Read the model definition and answer for the solid it produces. Units are mm, in the model's axes. A direction names the side the tool comes from. Coordinates: 2 decimals unless noted, no trailing zeros. Write each loop counter-clockwise with the first axis right and the second up, starting at its lowest first coordinate (ties: lowest second). Pieces come first, ordered by that corner, then holes. Notation, with made-up numbers: (48.25, -3) -> (90.25, -3) arc R18 ccw to (90.25, 3) -> close; hole circle Ø1 at (59.25, -24.5). An arc over 180 degrees is marked (long way). Write item = value, one per line. Start each with the question number.
1) Section B-B (z = 25.5) is taken. Count the separate pieces of the cut face and the enclosed holes in it, plus the area to 3 significant figures.
2) Section A-A (x = -6.5) is taken. Determine the outline of the cut face in (y, z), plus the area to 3 significant figures.
3) For a pull along Z with two mould halves and no side action, classify faces 6 (the face through (20.514, 15.136, 164.907)), 7 (the face through (0, -2, 10)), 8 (the face through (20.514, 16.424, 178.678)), 9 (the face through (9.25, 31.99, 138.16)) as released by +Z, released by -Z, zero draft, split by the parting line, or undercut.
4) Flat-ended cylindrical pins translate along their axes: pin 1 Ø2 at (x, z) = (-20, 9) entering from +Y; pin 2 Ø1 at (y, z) = (17, 173.5) entering from -X; pin 3 Ø2 at (x, z) = (-9, 95.5) entering from -Y; pin 4 Ø6 at (y, z) = (26.5, 143) entering from +X. Find the tip coordinate at first contact, or state that the pin passes through.
5) Find the intervals of material crossed by line 1 along X through (y, z) = (30.7, 42.55); line 2 along Y through (x, z) = (-12.5, 16); line 3 along X through (y, z) = (9.5, 15), in increasing order. Write a range as from..to.
6) A tool of negligible diameter and unlimited length cuts with its end or side. For faces 1 (the face through (-20.514, 12.916, 159.812)), 2 (the face through (22.27, 4.46, 199.87)), 3 (the face through (20.51, 20.11, 81.98)), 4 (the face through (20, 4, 204.877)), 5 (the face through (-7.38, 31.99, 55.43)), from which of +Z, -Z, +X, -X, +Y, -Y can it reach the whole face along a straight path? Write none if from no direction.
from build123d import *

# Parameters (mm, degrees)
SKETCH1_W                                 = 4
SKETCH1_H                                 = 1.4
SKETCH1_W_2                               = 39
SKETCH1_H_2                               = 2
SKETCH1_W_3                               = 2
SKETCH1_H_3                               = 27.8
SKETCH1_W_4                               = 19.5
BOSS_EXTRUDE1_DEPTH                       = 195
CUT_EXTRUDE1_DEPTH                        = 203.393181703
CUT_EXTRUDE1_DEPTH_BACK                   = 203.393181703
SKETCH2_W                                 = 191
SKETCH2_H                                 = 24
SKETCH3_W                                 = 29
SKETCH3_H                                 = 223
CUT_EXTRUDE2_DEPTH                        = 2
SKETCH5_W                                 = 45.8
SKETCH5_H                                 = 4
BOSS_EXTRUDE2_DEPTH                       = 2
SKETCH8_W                                 = 15
SKETCH8_H                                 = 8
BOSS_EXTRUDE4_DEPTH                       = 2
SKETCH9_W                                 = 15
SKETCH9_H                                 = 8
BOSS_EXTRUDE5_DEPTH                       = 2
BOSS_EXTRUDE6_DEPTH                       = 2
SKETCH6_W                                 = 45.8
SKETCH6_H                                 = 2.4
BOSS_EXTRUDE9_DEPTH                       = 19
SKETCH14_R                                = 4.7
SKETCH14_R_2                              = 1.6
CUT_EXTRUDE3_DEPTH                        = 19
TAP_DRILL_FOR_M3X0_5_TAP1_D               = 2.8
TAP_DRILL_FOR_M3X0_5_TAP1_DEPTH           = 10
TAP_DRILL_FOR_M3X0_5_TAP1_TIP             = 0.841204867
TAP_DRILL_FOR_M3X0_5_TAP1_ON_FACE_2_D     = 2.8
TAP_DRILL_FOR_M3X0_5_TAP1_ON_FACE_2_DEPTH = 10
TAP_DRILL_FOR_M3X0_5_TAP1_ON_FACE_2_TIP   = 0.841204867
TAP_DRILL_FOR_M3X0_5_TAP2_D               = 2.8
TAP_DRILL_FOR_M3X0_5_TAP2_DEPTH           = 10
TAP_DRILL_FOR_M3X0_5_TAP2_TIP             = 0.841204867
BOSS_EXTRUDE10_DEPTH                      = 2
BOSS_EXTRUDE11_START                      = -21.5
BOSS_EXTRUDE11_DEPTH                      = 43
BOSS_EXTRUDE12_DEPTH                      = 3
BOSS_EXTRUDE12_DEPTH_BACK                 = 1
SKETCH23_W                                = 36
SKETCH23_H                                = 20
FILLET3_R                                 = 3
FILLET4_R                                 = 3
FILLET5_R                                 = 3
FILLET6_R                                 = 3
CHAMFER3_SIZE                             = 8
CHAMFER3_SIZE_2                           = 1.410615846
BOSS_EXTRUDE14_DEPTH                      = 10
BOSS_EXTRUDE15_DEPTH                      = 10
FILLET7_R                                 = 2
CUT_EXTRUDE6_DEPTH                        = 10
CUT_EXTRUDE6_DEPTH_BACK                   = 10
SKETCH28_W                                = 29
SKETCH28_H                                = 20
CUT_EXTRUDE7_DEPTH                        = 2


# Read off the part's stored shape, not the designer's step: Boss-Extrude11
# Some blends are built 0.0001 mm under size
with BuildPart() as part:
    # Sketch1 → Boss-Extrude1 (new body)
    with BuildSketch(Plane.XY):
        Polygon((19.5, 1), (19.5, -1), (21.5, -1), (21.5, 5.2), (19.5, 5.2), (19.5, 3.8), align=None)
        with Locations((17.5, 4.5)):
            Rectangle(SKETCH1_W, SKETCH1_H)
        Rectangle(SKETCH1_W_2, SKETCH1_H_2)
        Polygon((-21.5, -1), (-19.5, -1), (-19.5, 1), (-19.5, 3.8), (-19.5, 5.2), (-21.5, 5.2), align=None)
        with Locations((-17.5, 4.5)):
            Rectangle(SKETCH1_W, SKETCH1_H)
        with Locations((20.5, 19.1)):
            Rectangle(SKETCH1_W_3, SKETCH1_H_3)
        with Locations((9.75, 32)):
            Rectangle(SKETCH1_W_4, SKETCH1_H_2)
        with Locations((-9.75, 32)):
            Rectangle(SKETCH1_W_4, SKETCH1_H_2)
        Polygon((-21.5, 33), (-21.5, 5.2), (-19.5, 5.2), (-19.5, 31), (-19.5, 33), align=None)
    extrude(amount=BOSS_EXTRUDE1_DEPTH)

    # Sketch2 → Cut-Extrude1 (cut, two sides: drawn at the far end of the back side and taken through both)
    with BuildSketch(Plane(origin=(21.5, 0, 0), x_dir=(0, 0, -1), z_dir=(1, 0, 0)).offset(-CUT_EXTRUDE1_DEPTH_BACK)):
        with Locations((-99.5, 19)):
            Rectangle(SKETCH2_W, SKETCH2_H)
    extrude(amount=CUT_EXTRUDE1_DEPTH + CUT_EXTRUDE1_DEPTH_BACK, mode=Mode.SUBTRACT)

    # Sketch3 → Cut-Extrude2 (cut)
    with BuildSketch(Plane(origin=(0, -1, 0), x_dir=(-1, 0, 0), z_dir=(0, -1, 0))):
        with Locations((0, -103.5)):
            Rectangle(SKETCH3_W, SKETCH3_H)
    extrude(amount=-CUT_EXTRUDE2_DEPTH, mode=Mode.SUBTRACT)

    # Sketch5 → Boss-Extrude2 (add)
    with BuildSketch(Plane(origin=(21.5, 0, 0), x_dir=(0, 0, -1), z_dir=(1, 0, 0))):
        with Locations((-22.9, 31)):
            Rectangle(SKETCH5_W, SKETCH5_H)
    extrude(amount=-BOSS_EXTRUDE2_DEPTH)

    # Sketch8 → Boss-Extrude4 (add)
    with BuildSketch(Plane(origin=(21.5, 0, 0), x_dir=(0, 0, -1), z_dir=(1, 0, 0))):
        with Locations((-11.5, 11)):
            Rectangle(SKETCH8_W, SKETCH8_H)
    extrude(amount=-BOSS_EXTRUDE4_DEPTH)

    # Sketch9 → Boss-Extrude5 (add)
    with BuildSketch(Plane.ZY.offset(21.5)):
        with Locations((11.5, 11)):
            Rectangle(SKETCH9_W, SKETCH9_H)
    extrude(amount=-BOSS_EXTRUDE5_DEPTH)

    # Sketch10 → Boss-Extrude6 (add)
    with BuildSketch(Plane.ZY.offset(21.5)):
        Polygon((4, 31), (146.749133454, 7), (195, 7), (52.250866546, 31), align=None)
        Polygon((195, 31), (52.250866546, 7), (4, 7), (146.749133454, 31), align=None)
    extrude(amount=-BOSS_EXTRUDE6_DEPTH)

    # Sketch6 → Boss-Extrude9 (add)
    with BuildSketch(Plane(origin=(21.5, 0, 0), x_dir=(0, 0, -1), z_dir=(1, 0, 0))):
        with Locations((-22.9, 30.2)):
            Rectangle(SKETCH6_W, SKETCH6_H)
    extrude(amount=BOSS_EXTRUDE9_DEPTH)

    # Sketch14 → Cut-Extrude3 (cut)
    with BuildSketch(Plane(origin=(0, 29, 0), x_dir=(-1, 0, 0), z_dir=(0, -1, 0))):
        with Locations(Location((-29.082681436, -25.05, 0), (0, 0, 90))):
            Circle(SKETCH14_R)
        with Locations(Location((-36.882681436, -42.55, 0), (0, 0, 90))):
            Circle(SKETCH14_R_2)
        with Locations(Location((-36.882681436, -7.55, 0), (0, 0, 90))):
            Circle(SKETCH14_R_2)
    extrude(amount=-CUT_EXTRUDE3_DEPTH, mode=Mode.SUBTRACT)

    # Tap Drill for M3x0.5 Tap1
    with Locations(Plane(origin=(-21.5, 9, 9.5), x_dir=(0, 0, -1), z_dir=(-1, 0, 0))):
        with Locations((0, 0)):
            Hole(TAP_DRILL_FOR_M3X0_5_TAP1_D / 2, depth=TAP_DRILL_FOR_M3X0_5_TAP1_DEPTH)
            with Locations((0, 0, -(TAP_DRILL_FOR_M3X0_5_TAP1_DEPTH + TAP_DRILL_FOR_M3X0_5_TAP1_TIP / 2))):  # 118° drill point
                Cone(0, TAP_DRILL_FOR_M3X0_5_TAP1_D / 2, TAP_DRILL_FOR_M3X0_5_TAP1_TIP, mode=Mode.SUBTRACT)

    # Tap Drill for M3x0.5 Tap1 on face 2
    with Locations(Plane(origin=(21.5, 9, 9.5), x_dir=(0, 0, 1), z_dir=(1, 0, 0))):
        with Locations((0, 0)):
            Hole(TAP_DRILL_FOR_M3X0_5_TAP1_ON_FACE_2_D / 2, depth=TAP_DRILL_FOR_M3X0_5_TAP1_ON_FACE_2_DEPTH)
            with Locations((0, 0, -(TAP_DRILL_FOR_M3X0_5_TAP1_ON_FACE_2_DEPTH + TAP_DRILL_FOR_M3X0_5_TAP1_ON_FACE_2_TIP / 2))):  # 118° drill point
                Cone(0, TAP_DRILL_FOR_M3X0_5_TAP1_ON_FACE_2_D / 2, TAP_DRILL_FOR_M3X0_5_TAP1_ON_FACE_2_TIP, mode=Mode.SUBTRACT)

    # Tap Drill for M3x0.5 Tap2
    with Locations(Plane(origin=(15, 33, 6), x_dir=(0, 0, 1), z_dir=(0, 1, 0))):
        with Locations((0, 0), (0, -30)):
            Hole(TAP_DRILL_FOR_M3X0_5_TAP2_D / 2, depth=TAP_DRILL_FOR_M3X0_5_TAP2_DEPTH)
            with Locations((0, 0, -(TAP_DRILL_FOR_M3X0_5_TAP2_DEPTH + TAP_DRILL_FOR_M3X0_5_TAP2_TIP / 2))):  # 118° drill point
                Cone(0, TAP_DRILL_FOR_M3X0_5_TAP2_D / 2, TAP_DRILL_FOR_M3X0_5_TAP2_TIP, mode=Mode.SUBTRACT)

    # Sketch13 → Boss-Extrude10 (add)
    with BuildSketch(Plane(origin=(21.5, 0, 0), x_dir=(0, 0, -1), z_dir=(1, 0, 0))):
        Polygon((-150.414335828, 23.503940905), (-162.805864398, 25.587292856), (-195, 7), (-179, 7), align=None)
        Polygon((-146.749133454, 31), (-195, 31), (-162.805864398, 25.587292856), (-146.805864398, 25.587292856), (-150.414335828, 23.503940905), (-52.250866546, 7), (-19, 7), (-19, 9.521906727), align=None)
        Polygon((-146.805864398, 25.587292856), (-162.805864398, 25.587292856), (-150.414335828, 23.503940905), align=None)
    extrude(amount=-BOSS_EXTRUDE10_DEPTH)

    # Boss-Extrude11 outline → Boss-Extrude11 (add)
    with BuildSketch(Plane.YZ.offset(BOSS_EXTRUDE11_START)):
        Polygon((32.658001311, 204.861593768), (31, 195), (33, 195), (34.658001311, 204.861593768), align=None)
    extrude(amount=BOSS_EXTRUDE11_DEPTH)

    # Sketch23 → Boss-Extrude12 (add, two sides: drawn at the far end of the back side and taken through both)
    with BuildSketch(Plane(origin=(0, -1, 0), x_dir=(-1, 0, 0), z_dir=(0, -1, 0)).offset(-BOSS_EXTRUDE12_DEPTH_BACK)):
        with Locations((0, -10)):
            Rectangle(SKETCH23_W, SKETCH23_H)
    extrude(amount=BOSS_EXTRUDE12_DEPTH + BOSS_EXTRUDE12_DEPTH_BACK)

    # Fillet3
    fillet3_edges = [part.edges().sort_by_distance(p)[0] for p in [
        (18, -4, 10),
        (0, -4, 20),
        (-18, -4, 10),
    ]]
    fillet(fillet3_edges, radius=FILLET3_R - 0.0001)  # a hair under: the kernel refuses the full size

    # Fillet4
    fillet4_edges = [part.edges().sort_by_distance(p)[0] for p in [
        (21.5, -1, 97.5),
        (-21.5, -1, 97.5),
    ]]
    fillet(fillet4_edges, radius=FILLET4_R)

    # Fillet5
    fillet5_edges = [part.edges().sort_by_distance(p)[0] for p in [
        (20.5, 15, 19),
        (-20.5, 15, 19),
    ]]
    fillet(fillet5_edges, radius=FILLET5_R)

    # Fillet6
    fillet6_edges = [part.edges().sort_by_distance(p)[0] for p in [
        (40.5, 30.2, 45.8),
        (40.5, 30.2, 0),
    ]]
    fillet(fillet6_edges, radius=FILLET6_R)

    # Chamfer3
    # the kernel refuses this chamfer: 8, 1.410615846 mm, written as the material it takes off along each edge
    with BuildSketch(Plane(origin=(14.5, 0, 20), x_dir=(0, 0.0066825316561017496, -0.9999776716360547), z_dir=(-1, 0, 0))) as chamfer3_piece_1:
        Polygon((CHAMFER3_SIZE * 0.999977671636, CHAMFER3_SIZE * 0.0066825316561), (-CHAMFER3_SIZE_2 * 0.00668253165453, CHAMFER3_SIZE_2 * 0.999977671401), (0, 0), align=None)
    extrude(amount=29, mode=Mode.SUBTRACT)

    # Sketch24 → Boss-Extrude14 (add, along a direction that is not the sketch's normal)
    with BuildSketch(Plane.XY.offset(195)):
        with BuildLine():
            Line((-21.5, 7), (-21.5, 2))
            ThreePointArc((-21.5, 2), (-20.621320344, -0.121320344), (-18.5, -1))
            Line((-18.5, -1), (-14.5, -1))
            Line((-14.5, -1), (-14.5, 1))
            Line((-14.5, 1), (-19.5, 1))
            Line((-19.5, 1), (-19.5, 3.8))
            Line((-19.5, 3.8), (-15.5, 3.8))
            Line((-15.5, 3.8), (-15.5, 5.2))
            Line((-15.5, 5.2), (-19.5, 5.2))
            Line((-19.5, 5.2), (-19.5, 7))
            Line((-19.5, 7), (-21.5, 7))
        make_face()
    extrude(amount=BOSS_EXTRUDE14_DEPTH, dir=(-0.15643446504023106, 0, 0.9876883405951378))

    # Sketch26 → Boss-Extrude15 (add, along a direction that is not the sketch's normal)
    with BuildSketch(Plane.XY.offset(195)):
        with BuildLine():
            Line((14.5, -1), (18.5, -1))
            ThreePointArc((18.5, -1), (20.621320344, -0.121320344), (21.5, 2))
            Line((21.5, 2), (21.5, 7))
            Line((21.5, 7), (19.5, 7))
            Line((19.5, 7), (19.5, 5.2))
            Line((19.5, 5.2), (15.5, 5.2))
            Line((15.5, 5.2), (15.5, 3.8))
            Line((15.5, 3.8), (19.5, 3.8))
            Line((19.5, 3.8), (19.5, 1))
            Line((19.5, 1), (14.5, 1))
            Line((14.5, 1), (14.5, -1))
        make_face()
    extrude(amount=BOSS_EXTRUDE15_DEPTH, dir=(0.15643446504022418, 0, 0.9876883405951389))

    # Fillet7
    fillet7_edges = [part.edges().sort_by_distance(p)[0] for p in [
        (21.5, 33, 97.5),
        (-21.5, 33, 97.5),
    ]]
    fillet(fillet7_edges, radius=FILLET7_R - 0.0001)  # a hair under: the kernel refuses the full size

    # Sketch27 → Cut-Extrude6 (cut, two sides: drawn at the far end of the back side and taken through both)
    with BuildSketch(Plane(origin=(0, 33, 0), x_dir=(1, 0, 0), z_dir=(0, 1, 0)).offset(-CUT_EXTRUDE6_DEPTH_BACK)):
        Polygon((4.150405868, -112.780977824), (14.5, -164.267549777), (14.5, -61.683054851), align=None)
        Polygon((-14.5, -163.178538917), (-4.150405868, -112.080615944), (-14.5, -60.594043992), align=None)
        Polygon((-12.502590183, -195), (12.517667731, -195), (0.054934327, -133.001103045), align=None)
        Polygon((-8.142372311, -204.861593768), (14.5, -204.861593768), (12.517667731, -195), (-12.502590183, -195), (-14.5, -204.861593768), align=None)
        Polygon((-14.5, -20), (-0.054934327, -91.860490724), (14.5, -20), align=None)
    extrude(amount=CUT_EXTRUDE6_DEPTH + CUT_EXTRUDE6_DEPTH_BACK, mode=Mode.SUBTRACT)

    # Sketch28 → Cut-Extrude7 (cut)
    with BuildSketch(Plane(origin=(0, 0, 0), x_dir=(1, 0, 0), z_dir=(0, 1, 0))):
        with Locations((0, -10)):
            Rectangle(SKETCH28_W, SKETCH28_H)
    extrude(amount=-CUT_EXTRUDE7_DEPTH, mode=Mode.SUBTRACT)


solid = part.part
Answer key:
q1.separate_pieces = 5
q1.enclosed_holes = 0
q1.area = 139 mm^2
q2.outline = (-4, 0) -> (-2, 0) -> (-2, 19.83) arc R3 ccw to (-4, 17) -> close; (31, 0) -> (33, 0) -> (33, 20) -> (31, 20) -> close; (31, 59.8) -> (33, 59.8) -> (33, 100.39) -> (31, 100.39) -> close; (31, 123.68) -> (33, 123.68) -> (33, 165.36) -> (31, 165.36) -> close
q2.area = 243 mm^2
q3.face_6 = undercut
q3.face_7 = zero draft
q3.face_8 = released by +Z
q3.face_9 = undercut
q4.pin_1 = 33
q4.pin_2 = 19.5
q4.pin_3 = through
q4.pin_4 = 21.5
q5.line_1 = -21.5..-19.5, 19.5..35.28, 38.48..40.5
q5.line_2 = -4..-2, 31..33
q5.line_3 = -21.5..-19.5, 19.5..21.5
q6.face_1 = +Z, -X
q6.face_2 = -Z, +X, +Y, -Y
q6.face_3 = +X
q6.face_4 = +Z, +X, -X, +Y, -Y
q6.face_5 = +Y, -Y
